```python
from build123d import *

# Parameters (mm, degrees)
BOSS_EXTRUDE1_DEPTH    = 26.35
CUT_EXTRUDE1_DEPTH     = 20
CUT_EXTRUDE3_START     = -26.35
CUT_EXTRUDE3_OUTLINE_R = 2.69253261
CUT_EXTRUDE3_DEPTH     = 26.35


# Read off the part's stored shape, not the designer's step: Cut-Extrude3
with BuildPart() as part:
    # Sketch1 → Boss-Extrude1 (new body)
    with BuildSketch(Plane(origin=(0, 0, 0), x_dir=(0, 0, -1), z_dir=(1, 0, 0))):
        with BuildLine():
            Line((19.05, 62.611), (-19.05, 62.611))
            ThreePointArc((-19.05, 62.611), (-36.688219036, 59.891543079), (-52.688239169, 51.985749479))
            Line((-52.688239169, 51.985749479), (-97.140382944, 20.791361801))
            ThreePointArc((-97.140382944, 20.791361801), (-107.949982522, -0.029797308), (-97.091561196, -20.82553716))
            Line((-97.091561196, -20.82553716), (-52.170359894, -52.19204611))
            ThreePointArc((-52.170359894, -52.19204611), (-36.41024798, -59.944824567), (-19.05, -62.611))
            Line((-19.05, -62.611), (19.05, -62.611))
            ThreePointArc((19.05, -62.611), (36.41024798, -59.944824567), (52.170359894, -52.19204611))
            Line((52.170359894, -52.19204611), (97.091561196, -20.82553716))
            ThreePointArc((97.091561196, -20.82553716), (107.949982522, -0.029797308), (97.140382944, 20.791361801))
            Line((97.140382944, 20.791361801), (52.688239169, 51.985749479))
            ThreePointArc((52.688239169, 51.985749479), (36.688219036, 59.891543079), (19.05, 62.611))
        make_face()
    extrude(amount=BOSS_EXTRUDE1_DEPTH)

    # Sketch2 → Cut-Extrude1 (cut)
    with BuildSketch(Plane(origin=(26.35, 0, 0), x_dir=(0, 0, -1), z_dir=(1, 0, 0))):
        with BuildLine():
            Line((19.05, 47.371), (-19.05, 47.371))
            ThreePointArc((-19.05, 47.371), (-32.09793649, 45.359271881), (-43.934009402, 39.510932398))
            Line((-43.934009402, 39.510932398), (-88.386153178, 8.31654472))
            ThreePointArc((-88.386153178, 8.31654472), (-92.709993009, -0.011918923), (-88.366624478, -8.330214864))
            Line((-88.366624478, -8.330214864), (-43.445423176, -39.696723814))
            ThreePointArc((-43.445423176, -39.696723814), (-31.837016725, -45.407178406), (-19.05, -47.371))
            Line((-19.05, -47.371), (19.05, -47.371))
            ThreePointArc((19.05, -47.371), (31.837016725, -45.407178406), (43.445423176, -39.696723814))
            Line((43.445423176, -39.696723814), (88.366624478, -8.330214864))
            ThreePointArc((88.366624478, -8.330214864), (92.709993009, -0.011918923), (88.386153178, 8.31654472))
            Line((88.386153178, 8.31654472), (43.934009402, 39.510932398))
            ThreePointArc((43.934009402, 39.510932398), (32.09793649, 45.359271881), (19.05, 47.371))
        make_face()
    extrude(amount=-CUT_EXTRUDE1_DEPTH, mode=Mode.SUBTRACT)

    # Cut-Extrude3 outline → Cut-Extrude3 (cut)
    with BuildSketch(Plane(origin=(26.35, 0, 0), x_dir=(0, 0, -1), z_dir=(1, 0, 0)).offset(CUT_EXTRUDE3_START)):
        with Locations((0, 54.991)):
            Circle(CUT_EXTRUDE3_OUTLINE_R)
        with Locations((20.828, 54.959960993)):
            Circle(CUT_EXTRUDE3_OUTLINE_R)
        with Locations((41.055062572, 49.992917233)):
            Circle(CUT_EXTRUDE3_OUTLINE_R)
        with Locations((58.492960359, 38.603215535)):
            Circle(CUT_EXTRUDE3_OUTLINE_R)
        with Locations((75.541877036, 26.639101521)):
            Circle(CUT_EXTRUDE3_OUTLINE_R)
        with Locations((92.763268061, 14.553953261)):
            Circle(CUT_EXTRUDE3_OUTLINE_R)
        with Locations((100.329987765, -0.020858116)):
            Circle(CUT_EXTRUDE3_OUTLINE_R)
        with Locations((92.763268061, -14.553953261)):
            Circle(CUT_EXTRUDE3_OUTLINE_R)
        with Locations((-20.828, 54.959960993)):
            Circle(CUT_EXTRUDE3_OUTLINE_R)
        with Locations((-41.055062572, 49.992917233)):
            Circle(CUT_EXTRUDE3_OUTLINE_R)
        with Locations((-58.492960359, 38.603215535)):
            Circle(CUT_EXTRUDE3_OUTLINE_R)
        with Locations((-75.541877036, 26.639101521)):
            Circle(CUT_EXTRUDE3_OUTLINE_R)
        with Locations((-92.763268061, 14.553953261)):
            Circle(CUT_EXTRUDE3_OUTLINE_R)
        with Locations((-100.329987765, -0.020858116)):
            Circle(CUT_EXTRUDE3_OUTLINE_R)
        with Locations((-92.763268061, -14.553953261)):
            Circle(CUT_EXTRUDE3_OUTLINE_R)
        with Locations((-75.541877036, -26.639101521)):
            Circle(CUT_EXTRUDE3_OUTLINE_R)
        with Locations((-58.492960359, -38.603215535)):
            Circle(CUT_EXTRUDE3_OUTLINE_R)
        with Locations((-41.055062572, -49.992917233)):
            Circle(CUT_EXTRUDE3_OUTLINE_R)
        with Locations((-20.828, -54.959960993)):
            Circle(CUT_EXTRUDE3_OUTLINE_R)
        with Locations((0, -54.991)):
            Circle(CUT_EXTRUDE3_OUTLINE_R)
        with Locations((20.828, -54.959960993)):
            Circle(CUT_EXTRUDE3_OUTLINE_R)
        with Locations((41.055062572, -49.992917233)):
            Circle(CUT_EXTRUDE3_OUTLINE_R)
        with Locations((58.492960359, -38.603215535)):
            Circle(CUT_EXTRUDE3_OUTLINE_R)
        with Locations((75.541877036, -26.639101521)):
            Circle(CUT_EXTRUDE3_OUTLINE_R)
    extrude(amount=CUT_EXTRUDE3_DEPTH, mode=Mode.SUBTRACT)


solid = part.part
```
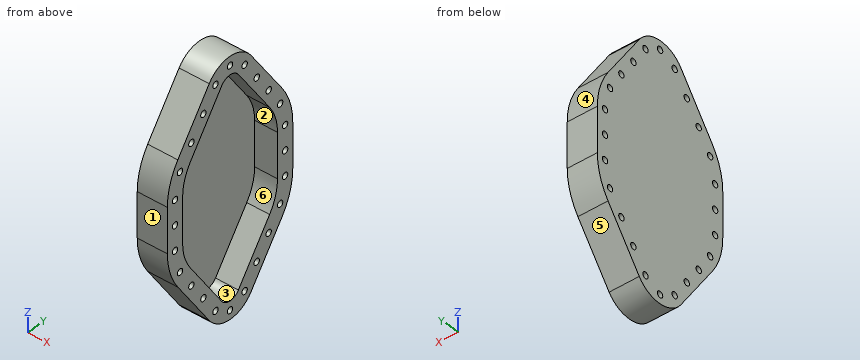
Geometry: final body of the model. Coordinates: model frame, mm. Face numbers are marked on the shaded views. A direction names the side the tool comes from. Round coordinates to 2 decimals unless told otherwise and drop trailing zeros. Order: outer loops, then holes, each group sorted by start corner. A loop starts at its lowest first (then second) coordinate and runs counter-clockwise, first axis right, second up. Notation, with made-up numbers: (71, 2.25) -> (103, 2.25) arc R9 cw to (103, 10.25) -> close; hole circle Ø4 at (-10.5, -20.5). An arc over 180 degrees is marked (long way). Use one line per item in the form item = value.
(1) Section D-D on x = 23.75. Count the separate pieces of the cut face and the enclosed holes in it, and give its area (3 significant figures).
Results list:
separate_pieces = 1
enclosed_holes = 25
area = 6,860 mm^2
(2) Section C-C on y = -45. Return loops of the section in (x, z).
Results list:
outline = (0, -62.47) -> (26.35, -62.47) -> (26.35, -33.07) -> (6.35, -33.07) -> (6.35, 33.07) -> (26.35, 33.07) -> (26.35, 62.47) -> (0, 62.47) -> close
(3) Access query for the marked faces 5 and 6. Directions: +Z, -Z, +X, -X, +Y, -Y. A direction counts if a zero-diameter tool reaches every point of the face in a straight line with its end or side. Return the directions, or none.
Results list:
face_5 = -Z, +X, -X, +Y
face_6 = +X
(4) Section B-B on z = 26.5. Return loops of the section in (x, y), and give its area (3 significant figures).
Results list:
outline = (0, -62.13) -> (26.35, -62.13) -> (26.35, -46.71) -> (6.35, -46.71) -> (6.35, 46.73) -> (26.35, 46.73) -> (26.35, 62.14) -> (0, 62.14) -> close
area = 1,410 mm^2
(5) Draft query along Z for the marked faces 1, 2, 3 and 4. Return one class per face: pulls with the +Z half, pulls with the -Z half, needs draft (parallel to the pull), parting line crosses it, or undercut.
Results list:
face_1 = needs draft
face_2 = undercut
face_3 = undercut
face_4 = pulls with the +Z half
(6) Section A-A on z = 0. Return loops of the section in (x, y).
Results list:
outline = (0, -62.61) -> (26.35, -62.61) -> (26.35, -57.68) -> (0, -57.68) -> close; (0, -52.3) -> (26.35, -52.3) -> (26.35, -47.37) -> (6.35, -47.37) -> (6.35, 47.37) -> (26.35, 47.37) -> (26.35, 52.3) -> (0, 52.3) -> close; (0, 57.68) -> (26.35, 57.68) -> (26.35, 62.61) -> (0, 62.61) -> close
(7) First-contact query: pin 1 Ø4.5 at (y, z) = (-49.99, 41.06) entering from +X; pin 2 Ø2 at (y, z) = (13, 11.5) entering from +X; pin 3 Ø6 at (x, z) = (9, 41) entering from +Y; pin 4 Ø2 at (x, y) = (19, -3) entering from +Z. Flat tips, straight axial feed; report the tip coordinate or a pass-through.
Results list:
pin_1 = through
pin_2 = 6.35
pin_3 = 59.46
pin_4 = 107.87
(8) Ray query, probe 1 along Y at (x, z) = (18.25, 0); probe 2 along Y at (x, z) = (3.75, -74); probe 3 along Z at (x, y) = (10, -38). Return the intervals inside material, ascending. Write a range as [from, to].
Results list:
probe_1 = [-62.61, -57.68], [-52.3, -47.37], [47.37, 52.3], [57.68, 62.61]
probe_2 = [-36.95, -28.85], [-24.43, 24.43], [28.85, 37.03]
probe_3 = [-72.5, -61.12], [-55.87, -45.88], [45.88, 55.87], [61.12, 72.5]
